```python
from build123d import *

# Parameters (mm, degrees)
SKETCH1_R               = 5.35
BOSS_EXTRUDE2_DEPTH     = 7
BOSS_EXTRUDE3_START     = 8
SKETCH3_R               = 5.35
BOSS_EXTRUDE3_DEPTH     = 8
BOSS_EXTRUDE4_DEPTH     = 3
CHAMFER1_SIZE           = 10
CHAMFER2_SIZE           = 5
CUT_EXTRUDE1_DEPTH      = 67.560662475
CUT_EXTRUDE1_DEPTH_BACK = 67.560662475
SKETCH5_W               = 31.474956737
SKETCH5_H               = 3.5
SKETCH5_H_2             = 8
CHAMFER3_SIZE           = 7
SKETCH6_R               = 11
BOSS_EXTRUDE5_DEPTH     = 5
SKETCH8_W               = 2.75
SKETCH8_H               = 7.59
SKETCH8_H_2             = 11.2
BOSS_EXTRUDE6_DEPTH     = 5
SKETCH9_R               = 3
BOSS_EXTRUDE7_DEPTH     = 72
CUT_EXTRUDE2_REACH      = 127.169
SKETCH10_W              = 8
SKETCH10_H              = 4
FILLET1_R               = 0.5


# Some blends are built 0.0001 mm under size
with BuildPart() as part:
    # Sketch1 → Boss-Extrude2 (new body)
    with BuildSketch(Plane.XY):
        Polygon((-19.503784034, -20), (19.503784034, -20), (19.503784034, -18.25), (62.978740771, -18.25), (62.978740771, 13), (19.503784034, 13), (19.503784034, 20), (-19.503784034, 20), align=None)
        Circle(SKETCH1_R, mode=Mode.SUBTRACT)
    extrude(amount=-BOSS_EXTRUDE2_DEPTH)

    # Sketch3 → Boss-Extrude3 (add)
    with BuildSketch(Plane.XY.offset(BOSS_EXTRUDE3_START)):
        with BuildLine():
            Line((7.668115805, 5.35), (62.978740771, 5.35))
            Line((62.978740771, 5.35), (62.978740771, 9.35))
            Line((62.978740771, 9.35), (0, 9.35))
            ThreePointArc((0, 9.35), (-9.35, 0), (0, -9.35))
            Line((0, -9.35), (62.978740771, -9.35))
            Line((62.978740771, -9.35), (62.978740771, -5.35))
            Line((62.978740771, -5.35), (7.668115805, -5.35))
            ThreePointArc((7.668115805, -5.35), (9.35, 0), (7.668115805, 5.35))
        make_face()
        Circle(SKETCH3_R, mode=Mode.SUBTRACT)
    extrude(amount=-BOSS_EXTRUDE3_DEPTH)

    # Sketch4 → Boss-Extrude4 (add)
    with BuildSketch(Plane.XY):
        with BuildLine():
            Line((0, -18.25), (62.978740771, -18.25))
            Line((62.978740771, -18.25), (62.978740771, -17.25))
            Line((62.978740771, -17.25), (8.306623863, -17.25))
            Line((8.306623863, -17.25), (0, -17.25))
            ThreePointArc((0, -17.25), (-17.25, 0), (0, 17.25))
            Line((0, 17.25), (0, 18.25))
            ThreePointArc((0, 18.25), (-18.25, 0), (0, -18.25))
        make_face()
    extrude(amount=BOSS_EXTRUDE4_DEPTH)

    # Chamfer1
    # the kernel refuses this chamfer: 10 mm, written as the material it takes off along each edge
    with BuildSketch(Plane(origin=(19.503784034, -20, 25.71682988), x_dir=(-0.9996219169112968, -0.027495876610586317, 0), z_dir=(0, 0, -1))) as chamfer1_piece_1_section:
        Polygon((CHAMFER1_SIZE * 0.999621916911, CHAMFER1_SIZE * 0.0274958766106), (-CHAMFER1_SIZE * 0.0274958766106, CHAMFER1_SIZE * 0.999621916911), (0, 0), align=None)
    chamfer1_piece_1 = extrude(amount=58.433659759, mode=Mode.PRIVATE)
    chamfer1_piece_1 = split(chamfer1_piece_1, bisect_by=Plane(origin=(14.814200223, -18.25, -3.5), z_dir=(0, -1, 0)), keep=Keep.TOP, mode=Mode.PRIVATE)
    add(chamfer1_piece_1, mode=Mode.SUBTRACT)

    # Chamfer2
    chamfer2_edges = [part.edges().sort_by_distance(p)[0] for p in [
        (-19.503784034, -20, -3.5),
        (-19.503784034, 20, -3.5),
    ]]
    chamfer(chamfer2_edges, length=CHAMFER2_SIZE)

    # Sketch5 → Cut-Extrude1 (cut, two sides: drawn at the far end of the back side and taken through both)
    with BuildSketch(Plane.XY.offset(-CUT_EXTRUDE1_DEPTH_BACK)):
        with Locations((40.241262403, 3.6)):
            Rectangle(SKETCH5_W, SKETCH5_H)
        with Locations((40.241262403, -7.15)):
            Rectangle(SKETCH5_W, SKETCH5_H_2)
    extrude(amount=CUT_EXTRUDE1_DEPTH + CUT_EXTRUDE1_DEPTH_BACK, mode=Mode.SUBTRACT)

    # Chamfer3
    chamfer3_edges = [part.edges().sort_by_distance(p)[0] for p in [
        (19.503784034, 20, -3.5),
    ]]
    chamfer(chamfer3_edges, length=CHAMFER3_SIZE - 0.0001)  # a hair under: the kernel refuses the full size


with BuildPart() as body_2:
    # Mirror9: mirrored copy
    add(part.part.mirror(Plane.XY.offset(-10)))

    # Sketch6 → Boss-Extrude5 (add)
    with BuildSketch(Plane.XY.offset(-13)):
        Circle(SKETCH6_R)
    extrude(amount=BOSS_EXTRUDE5_DEPTH)

    # Sketch8 → Boss-Extrude6 (add)
    with BuildSketch(Plane(origin=(62.978740771, 0, 0), x_dir=(0, 0, -1), z_dir=(1, 0, 0))):
        with Locations((16.5, 5.955)):
            Rectangle(SKETCH8_W, SKETCH8_H)
        with Locations((16.5, -8.9)):
            Rectangle(SKETCH8_W, SKETCH8_H_2)
    extrude(amount=BOSS_EXTRUDE6_DEPTH)

    # Sketch9 → Boss-Extrude7 (add)
    with BuildSketch(Plane(origin=(0, 0, -20), x_dir=(-1, 0, 0), z_dir=(0, 0, -1))):
        with Locations((-20.003784034, 0)):
            Circle(SKETCH9_R)
    extrude(amount=BOSS_EXTRUDE7_DEPTH)

    # Sketch10 → Cut-Extrude2 (cut, up to next)
    with BuildSketch(Plane(origin=(62.978740771, 0, 0), x_dir=(0, 0, -1), z_dir=(1, 0, 0)), mode=Mode.PRIVATE) as cut_extrude2_sk1:
        with Locations((24, -7.35)):
            Rectangle(SKETCH10_W, SKETCH10_H)
    cut_extrude2_tool1 = extrude(cut_extrude2_sk1.sketch, amount=-CUT_EXTRUDE2_REACH, mode=Mode.PRIVATE) & body_2.part
    add(cut_extrude2_tool1.solids().sort_by_distance((62.978741, -7.35, -24))[0], mode=Mode.SUBTRACT)

    # Fillet1
    fillet1_edges = [body_2.edges().sort_by_distance(p)[0] for p in [
        (0, 18.25, -21.5),
        (0, 17.25, -21.5),
    ]]
    fillet(fillet1_edges, radius=FILLET1_R - 0.0001)  # a hair under: the kernel refuses the full size


solid = body_2.part
```
The listing builds one solid part. Answer for the finished solid, in the listing's coordinates (mm). A direction names the side the tool comes from. Give positions to 0.01 mm unless a question says otherwise; leave off trailing zeros. Order: outer loops, then holes, each group sorted by start corner. A loop starts at its lowest first (then second) coordinate and runs counter-clockwise, first axis right, second up.
Item 1: The part is cut by section A-A, the plane y = 0. Give the vertices of the cut face in (x, z).
From the geometry:
outline: (-19.5, -20) - (-18.25, -20) - (-18.25, -23) - (-17.25, -23) - (-17.25, -20) - (-9.35, -20) - (-9.35, -28) - (-5.35, -28) - (-5.35, -13) - (5.35, -13) - (5.35, -28) - (9.35, -28) - (9.35, -20) - (17, -20) - (17, -92) - (23, -92) - (23, -20) - (62.98, -20) - (62.98, -13) - (11, -13) - (11, -8) - (-11, -8) - (-11, -13) - (-19.5, -13) - close
Item 2: For a pull along Y with two mould halves and no side action, classify faces 4 (the face through (67.979, 6, -16)), 5 (the face through (-18.25, 0.14, -21.48)), 6 (the face through (-17.039, -17.465, -16.549)), 7 (the face through (24.504, -7, -19)) as pulls with the +Y half, pulls with the -Y half, needs draft (parallel to the pull), parting line crosses it, or undercut.
From the geometry:
face 4: needs draft
face 5: parting line crosses it
face 6: pulls with the -Y half
face 7: undercut
Item 3: Which of the six approach directions +Z, -Z, +X, -X, +Y, -Y give full straight-line access (tool end or side, diameter ignored) to faces 1 (the face through (65, -14.5, -16)), 2 (the face through (40, 1.85, -16)), 3 (the face through (32, -17.25, -21))?
From the geometry:
face 1: +Z, -Z, +X, -Y
face 2: +Z, -Z
face 3: -Z, +X
Item 4: The part is cut by section C-C, the plane z = -47.5. Give the vertices of the cut face in (x, y), and give its area (3 significant figures).
From the geometry:
outline: circle Ø6 at (20, 0)
area: 28.3 mm2
Item 5: The part is cut by section D-D, the plane x = 15.5. Give the vertices of the cut face in (y, z), and give its area (3 significant figures).
From the geometry:
outline: (-18.25, -23) - (-17.25, -23) - (-17.25, -20) - (-9.35, -20) - (-9.35, -28) - (-5.35, -28) - (-5.35, -20) - (5.35, -20) - (5.35, -28) - (9.35, -28) - (9.35, -20) - (17, -20) - (17, -13) - (-18.25, -13) - close
area: 314 mm2
Item 6: Find the intervals of material crossed by probe 1 along Y at (x, z) = (0, -23.75); probe 2 along Y at (x, z) = (61.5, -22.5); probe 3 along Z at (x, y) = (2, -8.5), in increasing order.
From the geometry:
probe 1: y = -9.35 to -5.35, 5.35 to 9.35
probe 2: y = -18.25 to -17.25, 5.35 to 9.35
probe 3: z = -28 to -8
Item 7: Given pin 1 Ø6 at (y, z) = (5.5, -78) entering from +X; pin 2 Ø3 at (x, z) = (65, -16) entering from -Y; pin 3 Ø15 at (x, y) = (41, -2.5) entering from -Z, each flat-ended and moving along its own axis, determine where each tip first touches the part or whether it passes through.
From the geometry:
pin 1: stops at x = 21.66
pin 2: stops at y = -14.5
pin 3: stops at z = -20
Item 8: The part is cut by section B-B, the plane x = 58. Give the vertices of the cut face in (y, z), and give its area (3 significant figures).
From the geometry:
outline: (-18.25, -23) - (-17.25, -23) - (-17.25, -20) - (5.35, -20) - (5.35, -28) - (9.35, -28) - (9.35, -20) - (13, -20) - (13, -13) - (-18.25, -13) - close
area: 254 mm2
